```python
from build123d import *

# Parameters (mm, degrees)
THICKEN1_DEPTH      = 1
SKETCH6_W           = 3
SKETCH6_H           = 3
BOSS_EXTRUDE1_DEPTH = 10


# Read off the part's stored shape, not the designer's step: Thicken1
with BuildPart() as part:
    # Thicken1 outline → Thicken1 (new body)
    with BuildSketch(Plane.YZ):
        with BuildLine():
            add(Edge.make_bspline(
                [(10, -80), (41.657742077, -55.94021324), (47.197734967, -23.837728835), (10, 0)],
                knots=[0, 0, 0, 0, 1, 1, 1, 1], degree=3))
            Line((10, 0), (0, 0))
            Line((0, 0), (0, -80))
            Line((0, -80), (10, -80))
        make_face()
    extrude(amount=THICKEN1_DEPTH)

    # Sketch6 → Boss-Extrude1 (add)
    with BuildSketch(Plane.ZY):
        with Locations((-38.250665785, 1.5)):
            Rectangle(SKETCH6_W, SKETCH6_H)
    extrude(amount=BOSS_EXTRUDE1_DEPTH)


solid = part.part
```
Can you work these out from the model? Positions are in its coordinate system, mm. A direction names the side the tool comes from. Round coordinates to 2 decimals unless told otherwise and drop trailing zeros. Loops run counter-clockwise (first coordinate to the right, second up) from the corner with the lowest first, then second, coordinate; pieces in that order, holes last. Notation, with made-up numbers: M -31,60.25 L 18,60.25 A16 ccw 18,68.25 Z; hole C 72.25,-37 d6. An arc over 180 degrees is marked long. Answer as a JSON object with one key per item and string values. Group by question number.
Q1. Imagine slicing it at B-B, the plane y = 6. Please give me the cut outline in (x, z).
Q2. Please list where these lines run through material, in increasing order: L1, parallel to X at y = 9.5, z = -41.5; L2, parallel to Y at x = 0.75, z = -19.5; L3, parallel to Z at x = 0.5, y = 15.
Q3. On a 3-axis mill with a long thin cutter (end or side, diameter ignored), from which of +Z, -Z, +X, -X, +Y, -Y can I reach the whole of each face in a straight line? I mean faces 1 (the flat face through (-5, 1, -39.751)), 2 (the flat face through (-5, 1, -36.751)), 3 (the flat face through (-5, 3, -38)), 4 (the flat face through (0.4, 0, -39.8)). Say none if no direction works.
Q4. Imagine slicing it at A-A, the plane x = -5. Please give me the cut outline in (y, z).
Q5. Will these pins go through, and if not, where does the flat tip stop? pin 1 (1.5 mm diameter, centred on x = -4, z = -39, fed in from +Y); pin 2 (1.5 mm diameter, centred on x = -4, y = 1.5, fed in from -Z); pin 3 (2.5 mm diameter, centred on x = -3.5, y = 1.5, fed in from +Z); pin 4 (1.5 mm diameter, centred on x = -2, z = -35.5, fed in from -Y).
Findings:
{
 "1": {"outline": "M 0,-80 L 1,-80 L 1,0 L 0,0 Z"},
 "2": {"L1": "x = 0 to 1", "L2": "y = 0 to 30.35", "L3": "z = -75.95 to -3.44"},
 "3": {"face 1": "-Z, -X, +Y, -Y", "face 2": "+Z, -X, +Y, -Y", "face 3": "+Z, -Z, -X, +Y", "face 4": "+Z, -Z, +X, -X, -Y"},
 "4": {"outline": "M 0,-39.75 L 3,-39.75 L 3,-36.75 L 0,-36.75 Z"},
 "5": {"pin 1": "stops at y = 3", "pin 2": "stops at z = -39.75", "pin 3": "stops at z = -36.75", "pin 4": "passes through"}
}
